Read the model definition and answer for the solid it produces. Units are mm, in the model's axes. Round coordinates to 2 decimals unless told otherwise and drop trailing zeros. Write each loop counter-clockwise with the first axis right and the second up, starting at its lowest first coordinate (ties: lowest second). Pieces come first, ordered by that corner, then holes. Notation, with made-up numbers: M 26.25,-13.75 L 33.25,-13.75 A18 cw 33.25,21.25 Z; hole C 79,-19 d5. An arc over 180 degrees is marked long. Use one line per item in the form item = value. Start each with the question number.
```python
from build123d import *

# Parameters (mm, degrees)
F0_R     = 2.5
F1_DEPTH = 6.35


# Not quite as in the source:
# - a length typed as a fraction of an inch, garbled in the dataset ("3 / 203.2 mm" for 3/8 in), is restored


with BuildPart() as f1:
    # F0 (on Top) → F1 (new body)
    with BuildSketch(Plane.XY):
        with BuildLine():
            Line((-79.8226374756, -129.7651274337), (0, -197.3205080757))
            Line((0, -197.3205080757), (60, -197.3205080757))
            Line((60, -197.3205080757), (139.8226374756, -129.7651274337))
            ThreePointArc((139.8226374756, -129.7651274337), (177.2243186434, -85), (197.2912156208, -30.2266302477))
            Line((197.2912156208, -30.2266302477), (215.8845726812, 72.6794919243))
            Line((215.8845726812, 72.6794919243), (185.8845726812, 124.6410161514))
            Line((185.8845726812, 124.6410161514), (87.4685781451, 159.9917576814))
            ThreePointArc((87.4685781451, 159.9917576814), (30, 170), (-27.4685781451, 159.9917576814))
            Line((-27.4685781451, 159.9917576814), (-125.8845726812, 124.6410161514))
            Line((-125.8845726812, 124.6410161514), (-155.8845726812, 72.6794919243))
            Line((-155.8845726812, 72.6794919243), (-137.2912156208, -30.2266302477))
            ThreePointArc((-137.2912156208, -30.2266302477), (-117.2243186434, -85), (-79.8226374756, -129.7651274337))
        make_face()
        with Locations((10, -187.3205080757)):
            Circle(F0_R, mode=Mode.SUBTRACT)
        with Locations((50, -187.3205080757)):
            Circle(F0_R, mode=Mode.SUBTRACT)
        with Locations((-142.2243186434, 76.3397459622)):
            Circle(F0_R, mode=Mode.SUBTRACT)
        with Locations((-122.2243186434, 110.9807621135)):
            Circle(F0_R, mode=Mode.SUBTRACT)
        with Locations((202.2243186434, 76.3397459622)):
            Circle(F0_R, mode=Mode.SUBTRACT)
        with Locations((182.2243186434, 110.9807621135)):
            Circle(F0_R, mode=Mode.SUBTRACT)
    extrude(amount=F1_DEPTH)


solid = f1.part
```
Q1. Find section C-C on y = 21. Write down the section's boundary in (x, z), and give its area (3 significant figures).
Q2. Each of these flat-tipped pins is pushed along its axis until it touches: pin 1 Ø1.5 at (y, z) = (-123, 3.5) entering from +X; pin 2 Ø1 at (x, z) = (-35, 2.5) entering from -Y; pin 3 Ø3 at (x, z) = (-113, 3) entering from +Y. Where does it stop, or does it pass through?
Q3. Straight lines are drawn through the part: line 1 (Y direction, x = 29, z = 2.75); line 2 (Y direction, x = 186.5, z = 2.25); line 3 (X direction, y = 7.5, z = 0.5). For each, find the intervals that lie inside material, in ascending order. Write a range as [from, to].
Q4. Find section A-A on z = 4.75. Write down the section's boundary in (x, y).
Q5. Find section B-B on x = -71. Write down the section's boundary in (y, z), and give its area (3 significant figures).
Response:
q1.outline = M -146.55,0 L 206.55,0 L 206.55,6.35 L -146.55,6.35 Z
q1.area = 2,240 mm²
q2.pin_1 = 148.13
q2.pin_2 = -168.12
q2.pin_3 = 129.81
q3.line_1 = [-197.32, 170]
q3.line_2 = [-66.39, 123.58]
q3.line_3 = [-144.11, 204.11]
q4.outline = M -155.88,72.68 L -137.29,-30.23 A170 ccw -79.82,-129.77 L 0,-197.32 L 60,-197.32 L 139.82,-129.77 A170 ccw 197.29,-30.23 L 215.88,72.68 L 185.88,124.64 L 87.47,159.99 A170 ccw -27.47,159.99 L -125.88,124.64 Z; hole C -142.22,76.34 d5; hole C -122.22,110.98 d5; hole C 10,-187.32 d5; hole C 50,-187.32 d5; hole C 182.22,110.98 d5; hole C 202.22,76.34 d5
q5.outline = M -137.23,0 L 144.36,0 L 144.36,6.35 L -137.23,6.35 Z
q5.area = 1,790 mm²
